from build123d import *

# Parameters (mm, degrees)
SKETCH1_R           = 22.225
BOSS_EXTRUDE1_DEPTH = 31.75
SKETCH1_3_R         = 6.35
BOSS_EXTRUDE2_DEPTH = 19.05
CUT_EXTRUDE1_DEPTH  = 70.051688068


with BuildPart() as part:
    # Sketch1 → Boss-Extrude1 (new body)
    with BuildSketch(Plane.XY):
        Circle(SKETCH1_R)
    extrude(amount=BOSS_EXTRUDE1_DEPTH)

    # Sketch1<3> → Boss-Extrude2 (add)
    with BuildSketch(Plane.XY):
        with BuildLine():
            ThreePointArc((12.7, 44.45), (0, 57.15), (-12.7, 44.45))
            Line((-12.7, 44.45), (-12.7, 18.238986403))
            ThreePointArc((-12.7, 18.238986403), (0, 22.225), (12.7, 18.238986403))
            Line((12.7, 18.238986403), (12.7, 44.45))
        make_face()
        with Locations(Location((0, 44.45, 0), (0, 0, 180))):
            Circle(SKETCH1_3_R, mode=Mode.SUBTRACT)
    extrude(amount=BOSS_EXTRUDE2_DEPTH)

    # Sketch2 → Cut-Extrude1 (cut, through all)
    with BuildSketch(Plane.XY.offset(31.75)):
        with BuildLine():
            Line((0, 15.875), (0, -12.7))
            ThreePointArc((0, -12.7), (12.598777143, -1.600254515), (3.175, 12.296722124))
            Line((3.175, 12.296722124), (3.175, 15.875))
            Line((3.175, 15.875), (0, 15.875))
        make_face()
        with BuildLine():
            ThreePointArc((-3.175, 12.296722124), (-12.598777143, -1.600254515), (0, -12.7))
            Line((0, -12.7), (0, 15.875))
            Line((0, 15.875), (-3.175, 15.875))
            Line((-3.175, 15.875), (-3.175, 12.296722124))
        make_face()
    extrude(amount=-CUT_EXTRUDE1_DEPTH, mode=Mode.SUBTRACT)


solid = part.part
Geometry: final body of the model. Coordinates: model frame, mm. A direction names the side the tool comes from. Round coordinates to 2 decimals unless told otherwise and drop trailing zeros. Order: outer loops, then holes, each group sorted by start corner. A loop starts at its lowest first (then second) coordinate and runs counter-clockwise, first axis right, second up. Notation, with made-up numbers: (32, 64.25) - (49, 64.25) arc R11 cw to (49, 76.25) - close; hole circle Ø6 at (-3.75, 40.25). An arc over 180 degrees is marked (long way). Write each question's results on one line, items separated by ' | '.
Item 1: Material intervals for line 1 along Y through (x, z) = (0, 14.25) (3 decimals); line 2 along X through (y, z) = (44.45, 14.25); line 3 along Y through (x, z) = (-0.5, 20.5) (3 decimals), sorted ascending. Write a range as [from, to].
Completed:
line 1: [-22.225, -12.7], [15.875, 38.1], [50.8, 57.15] | line 2: [-12.7, -6.35], [6.35, 12.7] | line 3: [-22.219, -12.69], [15.875, 22.219]
Item 2: Reachability of faces 4 (the flat face through (-12.7, 32, 9)), 5 (the flat face through (12.7, 31, 9)), 6 (the flat face through (0, 15.875, 16)) from +Z, -Z, +X, -X, +Y, -Y: full face, straight path, thin tool, end or side. Return the list, or none.
Completed:
face 4: +Z, -Z, -X, +Y | face 5: +Z, -Z, +X, +Y | face 6: +Z, -Z
Item 3: First-contact query: pin 1 Ø8 at (x, z) = (-4.5, 11.5) entering from -Y; pin 2 Ø1.1 at (y, z) = (14.5, 15.5) entering from -X; pin 3 Ø1.1 at (y, z) = (15, 19.5) entering from +X; pin 4 Ø1 at (x, y) = (-13.5, 22.5) entering from +Z. Flat tips, straight axial feed; report the tip coordinate or a pass-through.
Completed:
pin 1: y = -22.22 | pin 2: x = -17.3 | pin 3: x = 16.89 | pin 4: through
Item 4: Section C-C, the plane z = 28. Return the cut outline in (x, y) (3 decimals), and give its area (3 significant figures).
Completed:
outline: circle Ø44.45 at (0, 0); hole (-3.175, 12.297) arc R12.7 ccw (long way) to (3.175, 12.297) - (3.175, 15.875) - (-3.175, 15.875) - close | area: 1,020 mm^2
Item 5: Mould query, pull axis Y, two halves, no side actions, for faces 1 (the cylindrical face through (0.279, 57.147, 9.392)), 2 (the flat face through (-3.175, 14, 16)), 3 (the cylindrical face through (-4.8, -21.7, 15.7)). Classes: pulls with the +Y half, pulls with the -Y half, needs draft (parallel to the pull), parting line crosses it, or undercut.
Completed:
face 1: pulls with the +Y half | face 2: undercut | face 3: parting line crosses it
Item 6: Section A-A, the plane y = 0. Return the cut outline in (x, z) (3 decimals).
Completed:
outline: (-22.225, 0) - (-12.7, 0) - (-12.7, 31.75) - (-22.225, 31.75) - close; (12.7, 0) - (22.225, 0) - (22.225, 31.75) - (12.7, 31.75) - close
Item 7: Section D-D, the plane y = 47.5. Return the cut outline in (x, z), and give its area (3 significant figures).
Completed:
outline: (-12.33, 0) - (-5.57, 0) - (-5.57, 19.05) - (-12.33, 19.05) - close; (5.57, 0) - (12.33, 0) - (12.33, 19.05) - (5.57, 19.05) - close | area: 258 mm^2
Item 8: Section B-B, the plane z = 14. Return the cut outline in (x, y) (3 decimals).
Completed:
outline: (-12.7, 18.239) arc R22.225 ccw (long way) to (12.7, 18.239) - (12.7, 44.45) arc R12.7 ccw to (-12.7, 44.45) - close; hole circle Ø12.7 at (0, 44.45); hole (-3.175, 12.297) arc R12.7 ccw (long way) to (3.175, 12.297) - (3.175, 15.875) - (-3.175, 15.875) - close
